Source: CAD feature listing. Evaluate the final solid. Frame: model axes, mm. A direction names the side the tool comes from. Give positions to 0.01 mm unless a question says otherwise; leave off trailing zeros. Order: outer loops, then holes, each group sorted by start corner. A loop starts at its lowest first (then second) coordinate and runs counter-clockwise, first axis right, second up.
from build123d import *

# Parameters (mm, degrees)
SKETCH1_W               = 230
SKETCH1_H               = 150
BOSS_EXTRUDE1_DEPTH     = 3.5
SKETCH4_R               = 8.5
SKETCH4_W               = 15.5
SKETCH4_H               = 16
CUT_EXTRUDE2_DEPTH      = 100
SKETCH2_W               = 230
SKETCH2_H               = 150
SKETCH2_W_2             = 220
SKETCH2_H_2             = 140
CUT_EXTRUDE3_DEPTH      = 1.5
SKETCH5_W               = 12
SKETCH5_H               = 12
SKETCH5_R               = 1.75
CUT_EXTRUDE4_DEPTH      = 1.5
SKETCH7_R               = 1.75
CUT_EXTRUDE5_DEPTH      = 10
MIRROR2_COPY_1_SKETCH_W = 12
MIRROR2_COPY_1_SKETCH_H = 12
MIRROR2_COPY_1_SKETCH_R = 1.75
MIRROR2_COPY_1_DEPTH    = 1.5
MIRROR2_COPY_2_SKETCH_R = 1.75
MIRROR2_COPY_2_DEPTH    = 10
SKETCH8_R               = 2.6
CUT_EXTRUDE6_DEPTH      = 10
SKETCH9_W               = 7
SKETCH9_H               = 7
CUT_EXTRUDE7_DEPTH      = 1


with BuildPart() as part:
    # Sketch1 → Boss-Extrude1 (new body)
    with BuildSketch(Plane(origin=(0, 0, 0), x_dir=(1, 0, 0), z_dir=(0, 1, 0))):
        Rectangle(SKETCH1_W, SKETCH1_H)
    extrude(amount=BOSS_EXTRUDE1_DEPTH)

    # Sketch4 → Cut-Extrude2 (cut)
    with BuildSketch(Plane.XZ):
        with Locations(Location((-75, -35, 0), (0, 0, 270))):
            Circle(SKETCH4_R)
        with Locations(Location((75, -35, 0), (0, 0, 90))):
            Circle(SKETCH4_R)
        with Locations((0, 5)):
            Rectangle(SKETCH4_W, SKETCH4_H)
    extrude(amount=-CUT_EXTRUDE2_DEPTH, mode=Mode.SUBTRACT)

    # Sketch2 → Cut-Extrude3 (cut)
    with BuildSketch(Plane(origin=(0, 3.5, 0), x_dir=(1, 0, 0), z_dir=(0, 1, 0))):
        Rectangle(SKETCH2_W, SKETCH2_H)
        Rectangle(SKETCH2_W_2, SKETCH2_H_2, mode=Mode.SUBTRACT)
    extrude(amount=-CUT_EXTRUDE3_DEPTH, mode=Mode.SUBTRACT)

    # Sketch5 → Cut-Extrude4 (cut)
    with BuildSketch(Plane(origin=(0, 3.5, 0), x_dir=(1, 0, 0), z_dir=(0, 1, 0))):
        with Locations((-104, 64)):
            Rectangle(SKETCH5_W, SKETCH5_H)
        with Locations(Location((-104.3, 64.3, 0), (0, 0, 270))):
            Circle(SKETCH5_R, mode=Mode.SUBTRACT)
    cut_extrude4 = extrude(amount=-CUT_EXTRUDE4_DEPTH, mode=Mode.SUBTRACT)

    # Sketch7 → Cut-Extrude5 (cut)
    with BuildSketch(Plane(origin=(0, 3.5, 0), x_dir=(1, 0, 0), z_dir=(0, 1, 0))):
        with Locations(Location((-104.3, 64.3, 0), (0, 0, 270))):
            Circle(SKETCH7_R)
    cut_extrude5 = extrude(amount=-CUT_EXTRUDE5_DEPTH, mode=Mode.SUBTRACT)

    # Mirror1: Cut-Extrude4, Cut-Extrude5 across plane
    add(cut_extrude4.mirror(Plane(origin=(0, 0, 0), x_dir=(0, 0, 1), z_dir=(1, 0, 0))), mode=Mode.SUBTRACT)
    add(cut_extrude5.mirror(Plane(origin=(0, 0, 0), x_dir=(0, 0, 1), z_dir=(1, 0, 0))), mode=Mode.SUBTRACT)

    # Mirror2: Cut-Extrude4, Cut-Extrude5 across plane
    add(cut_extrude4.mirror(Plane.XY), mode=Mode.SUBTRACT)
    add(cut_extrude5.mirror(Plane.XY), mode=Mode.SUBTRACT)

    # Mirror2 copy 1 sketch → Mirror2 copy 1 (cut)
    with BuildSketch(Plane(origin=(0, 3.5, 0), x_dir=(-1, 0, 0), z_dir=(0, 1, 0))):
        with Locations((-104, 64)):
            Rectangle(MIRROR2_COPY_1_SKETCH_W, MIRROR2_COPY_1_SKETCH_H)
        with Locations(Location((-104.3, 64.3, 0), (0, 0, 270))):
            Circle(MIRROR2_COPY_1_SKETCH_R, mode=Mode.SUBTRACT)
    extrude(amount=-MIRROR2_COPY_1_DEPTH, mode=Mode.SUBTRACT)

    # Mirror2 copy 2 sketch → Mirror2 copy 2 (cut)
    with BuildSketch(Plane(origin=(0, 3.5, 0), x_dir=(-1, 0, 0), z_dir=(0, 1, 0))):
        with Locations(Location((-104.3, 64.3, 0), (0, 0, 270))):
            Circle(MIRROR2_COPY_2_SKETCH_R)
    extrude(amount=-MIRROR2_COPY_2_DEPTH, mode=Mode.SUBTRACT)

    # Sketch8 → Cut-Extrude6 (cut)
    with BuildSketch(Plane.XZ):
        with BuildLine():
            ThreePointArc((-72.4, 55), (-75, 57.6), (-77.6, 55))
            Line((-77.6, 55), (-72.4, 55))
        make_face()
        with BuildLine():
            Line((-72.4, 55), (-77.6, 55))
            ThreePointArc((-77.6, 55), (-75, 52.4), (-72.4, 55))
        make_face()
        with Locations(Location((50, 55, 0), (0, 0, 270))):
            Circle(SKETCH8_R)
        with Locations(Location((65, 55, 0), (0, 0, 270))):
            Circle(SKETCH8_R)
        with Locations(Location((80, 55, 0), (0, 0, 270))):
            Circle(SKETCH8_R)
    extrude(amount=-CUT_EXTRUDE6_DEPTH, mode=Mode.SUBTRACT)

    # Sketch9 → Cut-Extrude7 (cut)
    with BuildSketch(Plane(origin=(0, 3.5, 0), x_dir=(1, 0, 0), z_dir=(0, 1, 0))):
        with Locations((0, 16)):
            Rectangle(SKETCH9_W, SKETCH9_H)
        with Locations((0, -26)):
            Rectangle(SKETCH9_W, SKETCH9_H)
    extrude(amount=-CUT_EXTRUDE7_DEPTH, mode=Mode.SUBTRACT)


solid = part.part
1) Pull-direction query (X, two-part tool) for faces 1 (the face through (81.757, 1.726, 56.916)), 2 (the face through (-1, 2, -73)); classes: +X half, -X half, draft (parallel to the pull), parting line (faces both ways), or undercut.
Checks:
face 1: undercut
face 2: draft
2) First-contact query: pin 1 Ø13.5 at (x, z) = (75, -35) entering from -Y; pin 2 Ø1.2 at (y, z) = (3, 9) entering from +X; pin 3 Ø0.8 at (x, y) = (102, 2.5) entering from -Z; pin 4 Ø1.1 at (x, y) = (-1, 3) entering from +Z. Flat tips, straight axial feed; report the tip coordinate or a pass-through.
Checks:
pin 1: passes through
pin 2: stops at x = 110
pin 3: stops at z = -58
pin 4: stops at z = 70
3) Ray query, L1, parallel to X at y = 2.85, z = 55; L2, parallel to Z at x = -104.3, y = 0.5; L3, parallel to Z at x = -2.5, y = 3.05. Return the intervals inside material, ascending.
Checks:
L1: x = -110 to -77.6, -72.4 to 47.4, 52.6 to 62.4, 67.6 to 77.4, 82.6 to 110
L2: z = -75 to -66.05, -62.55 to 62.55, 66.05 to 75
L3: z = -70 to -19.5, -12.5 to -3, 13 to 22.5, 29.5 to 70
4) Section query C-C on x = 50. Output: boundary loops of the cut face in (y, z).
Checks:
outline: (0, -75) - (2, -75) - (2, -70) - (3.5, -70) - (3.5, 52.4) - (0, 52.4) - close; (0, 57.6) - (3.5, 57.6) - (3.5, 70) - (2, 70) - (2, 75) - (0, 75) - close
5) Reachability of faces 3 (the face through (0, 2.5, 26)), 4 (the face through (-2, 3.5, 15)) from +Z, -Z, +X, -X, +Y, -Y: full face, straight path, thin tool, end or side. Return the list, or none.
Checks:
face 3: +Y
face 4: +Z, -Z, +X, -X, +Y
6) Section query B-B on y = 1. State how many separate pieces and enclosed holes the cut face has, and give its area (3 significant figures).
Checks:
separate pieces: 1
enclosed holes: 11
area: 33,700 mm2
7) Section query D-D on z = 3. Output: boundary loops of the cut face in (x, y).
Checks:
outline: (-115, 0) - (-7.75, 0) - (-7.75, 3.5) - (-110, 3.5) - (-110, 2) - (-115, 2) - close; (7.75, 0) - (115, 0) - (115, 2) - (110, 2) - (110, 3.5) - (7.75, 3.5) - close
8) Section query A-A on z = 55. Output: boundary loops of the cut face in (x, y), and give its area (3 significant figures).
Checks:
outline: (-115, 0) - (-77.6, 0) - (-77.6, 3.5) - (-110, 3.5) - (-110, 2) - (-115, 2) - close; (-72.4, 0) - (47.4, 0) - (47.4, 3.5) - (-72.4, 3.5) - close; (52.6, 0) - (62.4, 0) - (62.4, 3.5) - (52.6, 3.5) - close; (67.6, 0) - (77.4, 0) - (77.4, 3.5) - (67.6, 3.5) - close; (82.6, 0) - (115, 0) - (115, 2) - (110, 2) - (110, 3.5) - (82.6, 3.5) - close
area: 717 mm2
